from build123d import *

# Parameters (mm, degrees)
F1_DEPTH = 43
F2_R     = 14.8013323082
F4_DEPTH = 42.1
F3_R     = 10.3723176452
F5_DEPTH = 43.001


with BuildPart() as f1:
    # F0 (on Top) → F1 (new body)
    with BuildSketch(Plane.XY):
        with BuildLine():
            Line((17.0280970633, 0), (17.0280970633, 22.9404084384))
            Line((17.0280970633, 22.9404084384), (-17.0280970633, 22.9404084384))
            Line((-17.0280970633, 22.9404084384), (-17.0280970633, 0))
            ThreePointArc((-17.0280970633, 0), (0, -17.0280970633), (17.0280970633, 0))
        make_face()
    extrude(amount=F1_DEPTH)

    # F2 (on face) → F4 (cut)
    with BuildSketch(Plane.XY.offset(43)):
        Circle(F2_R)
    extrude(amount=-F4_DEPTH, mode=Mode.SUBTRACT)

    # F3 (on face) → F5 (cut, through all)
    with BuildSketch(Plane.XY.offset(43)):
        Circle(F3_R)
    extrude(amount=-F5_DEPTH, mode=Mode.SUBTRACT)


solid = f1.part
Design review of the part built by this model. Coordinates are the model's own, in mm. Coordinates: 2 decimals unless noted, no trailing zeros. Order: outer loops, then holes, each group sorted by start corner. A loop starts at its lowest first (then second) coordinate and runs counter-clockwise, first axis right, second up. Notation, with made-up numbers: (20.5, 72.5) - (62.5, 72.5) arc R24 cw to (62.5, 90.5) - close; hole circle Ø8 at (67, 47). An arc over 180 degrees is marked (long way). Put each result on its own line as item: value.
1) Insertion check: P1, Ø3, axis at x = -10.5, y = -1, coming from the +Z side. The pin has a flat end and moves straight along its axis. Give the tip position at first contact, or say it passes through.
Response values:
P1: stops at z = 0.9
2) Wall thickness on L1, parallel to Y at x = -0.5, z = 12; L2, parallel to Z at x = -10.5, y = -7; L3, parallel to Y at x = -1.5, z = 31: over which ranges is each line inside the solid? List them lowest first. Write a range as from..to.
Response values:
L1: y = -17.02..-14.79, 14.79..22.94
L2: z = 0..0.9
L3: y = -16.96..-14.73, 14.73..22.94
3) Take a section at B-B, the plane y = 1.5. Give the boundary of the cut face in (x, z).
Response values:
outline: (-17.03, 0) - (-10.26, 0) - (-10.26, 0.9) - (-14.73, 0.9) - (-14.73, 43) - (-17.03, 43) - close; (10.26, 0) - (17.03, 0) - (17.03, 43) - (14.73, 43) - (14.73, 0.9) - (10.26, 0.9) - close
4) Take a section at A-A, the plane x = 0. Give the boundary of the cut face in (y, z).
Response values:
outline: (-17.03, 0) - (-10.37, 0) - (-10.37, 0.9) - (-14.8, 0.9) - (-14.8, 43) - (-17.03, 43) - close; (10.37, 0) - (22.94, 0) - (22.94, 43) - (14.8, 43) - (14.8, 0.9) - (10.37, 0.9) - close
5) The part is to be moulded in two halves that separate along Y. For faces 1 (the face through (0, 22.94, 21)), 2 (the face through (17.028, 11, 21)), 3 (the face through (-3.21, -14.45, 22.24)), 4 (the face through (-10.1, -3.1, 0.9)), say which applies: released by +Y, released by -Y, zero draft, split by the parting line, or undercut.
Response values:
face 1: released by +Y
face 2: zero draft
face 3: undercut
face 4: undercut
6) Take a section at C-C, the plane z = 11.5. Give the boundary of the cut face in (x, y).
Response values:
outline: (-17.03, 0) arc R17.03 ccw to (17.03, 0) - (17.03, 22.94) - (-17.03, 22.94) - close; hole circle Ø29.6 at (0, 0)
7) Take a section at D-D, the plane x = 12. Give the boundary of the cut face in (y, z), and give its area (3 significant figures).
Response values:
outline: (-12.08, 0) - (22.94, 0) - (22.94, 43) - (8.66, 43) - (8.66, 0.9) - (-8.66, 0.9) - (-8.66, 43) - (-12.08, 43) - close
area: 776 mm²
